Source: CAD feature listing. Evaluate the final solid. Frame: model axes, mm. Face numbers are marked on the shaded views. A direction names the side the tool comes from. Give positions to 0.01 mm unless a question says otherwise; leave off trailing zeros. Write each loop counter-clockwise with the first axis right and the second up, starting at its lowest first coordinate (ties: lowest second). Pieces come first, ordered by that corner, then holes. Notation, with made-up numbers: (86.25, 89) -> (97.25, 89) arc R24 cw to (97.25, 116) -> close; hole circle Ø8 at (72.5, 14.25). An arc over 180 degrees is marked (long way). Answer as a JSON object with one key per item and string values. Group by question number.
Item 1: First-contact query: pin 1 Ø8 at (x, z) = (24.925, -6) entering from -Y; pin 2 Ø2.5 at (y, z) = (-22.225, -93.5) entering from +X; pin 3 Ø1 at (y, z) = (-12.5, -59) entering from +X. Flat tips, straight axial feed; report the tip coordinate or a pass-through.
Item 2: Section query A-A on z = -33.5. Return the cut outline in (x, y) (3 decimals), plus the area to 3 significant figures.
Item 3: Ray query, probe 1 along X at (y, z) = (1.15, -93.5) (3 decimals); probe 2 along Y at (x, z) = (-2.2, -93.5) (3 decimals); probe 3 along X at (y, z) = (-1, -86) (3 decimals). Return the intervals inside material, ascending. Write a range as from..to.
Item 4: Section query D-D on z = -78.5. Return the cut outline in (x, y) (3 decimals).
Item 5: Section query B-B on y = -16.5. Return the cut outline in (x, z) (3 decimals), plus the area to 3 significant figures.
Item 6: Access query for the marked faces 1 and 2. Directions: +Z, -Z, +X, -X, +Y, -Y. A direction counts if a zero-diameter tool reaches every point of the face in a straight line with its end or side. Return the directions, or none.
Item 7: Section query C-C on z = -6. Return the cut outline in (x, y) (3 decimals).
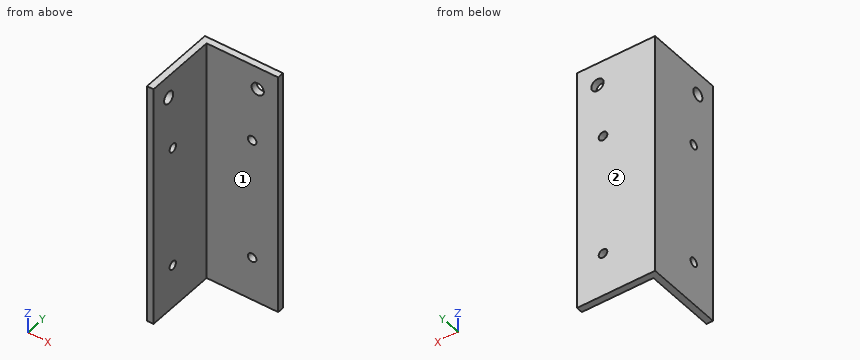
from build123d import *

# Parameters (mm, degrees)
SKETCH1_W                      = 38.1
SKETCH1_H                      = 120
BOSS_EXTRUDE1_DEPTH            = 38.1
SKETCH2_W                      = 34.925
SKETCH2_H                      = 34.925
CUT_EXTRUDE1_DEPTH             = 130.767142413
F_4_2_4_2_DIAMETER_HOLE1_D     = 4.2
F_6_0_6_DIAMETER_HOLE1_D       = 6
F_4_2_4_2_DIAMETER_HOLE2_D     = 4.2
F_4_2_4_2_DIAMETER_HOLE2_DEPTH = 38.1
F_6_0_6_DIAMETER_HOLE2_D       = 6
F_6_0_6_DIAMETER_HOLE2_DEPTH   = 38.1
F_6_0_6_DIAMETER_HOLE3_D       = 6
F_6_0_6_DIAMETER_HOLE3_DEPTH   = 38.1
F_4_2_4_2_DIAMETER_HOLE3_D     = 4.2
SKETCH15_R                     = 2.1
SKETCH15_R_2                   = 3
BOSS_EXTRUDE2_DEPTH            = 3.175
BOSS_EXTRUDE3_START            = -3.175
SKETCH16_R                     = 3
SKETCH16_R_2                   = 2.1
BOSS_EXTRUDE3_DEPTH            = 3.175


with BuildPart() as part:
    # Sketch1 → Boss-Extrude1 (new body)
    with BuildSketch(Plane.XZ.offset(34.925)):
        with Locations((15.875, -55)):
            Rectangle(SKETCH1_W, SKETCH1_H)
    extrude(amount=-BOSS_EXTRUDE1_DEPTH)

    # Sketch2 → Cut-Extrude1 (cut, through all)
    with BuildSketch(Plane(origin=(0, 0, -115), x_dir=(-1, 0, 0), z_dir=(0, 0, -1))):
        with Locations((-17.4625, -17.4625)):
            Rectangle(SKETCH2_W, SKETCH2_H)
    extrude(amount=-CUT_EXTRUDE1_DEPTH, mode=Mode.SUBTRACT)

    # Ø4.2 (4.2) Diameter Hole1 (through all)
    with Locations(Plane(origin=(0, 0, 0), x_dir=(-1, 0, 0), z_dir=(0, -1, 0))):
        with Locations((-5, 35.97), (-5, 91.03)):
            Hole(F_4_2_4_2_DIAMETER_HOLE1_D / 2)

    # Ø6.0 (6) Diameter Hole1 (through all)
    with Locations(Plane(origin=(0, 0, 0), x_dir=(-1, 0, 0), z_dir=(0, -1, 0))):
        with Locations((-22.225, 106.5), (-22.225, 46.5)):
            Hole(F_6_0_6_DIAMETER_HOLE1_D / 2)

    # Ø4.2 (4.2) Diameter Hole2
    with Locations(Plane(origin=(0, 3.175, 0), x_dir=(1, 0, 0), z_dir=(0, 1, 0))):
        with Locations((22.225, 33.5), (22.225, 93.5), (29.296067812, 100.571067812), (29.296067812, 26.428932188)):
            Hole(F_4_2_4_2_DIAMETER_HOLE2_D / 2, depth=F_4_2_4_2_DIAMETER_HOLE2_DEPTH)

    # Ø6.0 (6) Diameter Hole2
    with Locations(Plane(origin=(0, 3.175, 0), x_dir=(1, 0, 0), z_dir=(0, 1, 0))):
        with Locations((24.925, 6)):
            Hole(F_6_0_6_DIAMETER_HOLE2_D / 2, depth=F_6_0_6_DIAMETER_HOLE2_DEPTH)

    # Ø6.0 (6) Diameter Hole3
    with Locations(Plane.ZY.offset(3.175)):
        with Locations((-6, -24.925), (-106.5, -22.225), (-46.5, -22.225)):
            Hole(F_6_0_6_DIAMETER_HOLE3_D / 2, depth=F_6_0_6_DIAMETER_HOLE3_DEPTH)

    # Ø4.2 (4.2) Diameter Hole3 (through all)
    with Locations(Plane.ZY.offset(3.175)):
        with Locations((-93.5, -22.225), (-33.5, -22.225), (-35.97, -5), (-91.03, -5), (-100.571067812, -29.296067812), (-26.428932188, -29.296067812)):
            Hole(F_4_2_4_2_DIAMETER_HOLE3_D / 2)

    # Sketch15 → Boss-Extrude2 (add)
    with BuildSketch(Plane(origin=(0, 3.175, 0), x_dir=(1, 0, 0), z_dir=(0, 1, 0))):
        with Locations((29.296067812, 26.428932188)):
            Circle(SKETCH15_R)
        with Locations((29.296067812, 100.571067812)):
            Circle(SKETCH15_R)
        with Locations((22.225, 106.5)):
            Circle(SKETCH15_R_2)
        with Locations((22.225, 46.5)):
            Circle(SKETCH15_R_2)
        with Locations((5, 35.97)):
            Circle(SKETCH15_R)
        with Locations((5, 91.03)):
            Circle(SKETCH15_R)
    extrude(amount=-BOSS_EXTRUDE2_DEPTH)

    # Sketch16 → Boss-Extrude3 (add)
    with BuildSketch(Plane.ZY.offset(3.175).offset(BOSS_EXTRUDE3_START)):
        with Locations((-106.5, -22.225)):
            Circle(SKETCH16_R)
        with Locations((-100.571067812, -29.296067812)):
            Circle(SKETCH16_R_2)
        with Locations((-46.5, -22.225)):
            Circle(SKETCH16_R)
        with Locations((-26.428932188, -29.296067812)):
            Circle(SKETCH16_R_2)
        with Locations((-35.97, -5)):
            Circle(SKETCH16_R_2)
        with Locations((-91.03, -5)):
            Circle(SKETCH16_R_2)
    extrude(amount=BOSS_EXTRUDE3_DEPTH)


solid = part.part
Worked answers:
{
 "1": {"pin 1": "y = 0", "pin 2": "through", "pin 3": "x = 0"},
 "2": {"outline": "(-3.175, -34.925) -> (0, -34.925) -> (0, -24.325) -> (-3.175, -24.325) -> close; (-3.175, -20.125) -> (0, -20.125) -> (0, 0) -> (20.125, 0) -> (20.125, 3.175) -> (-3.175, 3.175) -> close; (24.325, 0) -> (34.925, 0) -> (34.925, 3.175) -> (24.325, 3.175) -> close", "area": "205 mm^2"},
 "3": {"probe 1": "-3.175..20.125, 24.325..34.925", "probe 2": "-34.925..-24.325, -20.125..3.175", "probe 3": "-3.175..0"},
 "4": {"outline": "(-3.175, -34.925) -> (0, -34.925) -> (0, 0) -> (34.925, 0) -> (34.925, 3.175) -> (-3.175, 3.175) -> close"},
 "5": {"outline": "(-3.175, -115) -> (0, -115) -> (0, 5) -> (-3.175, 5) -> close", "area": "381 mm^2"},
 "6": {"face 1": "+Z, -Z, +X, -Y", "face 2": "+Z, -Z, +X, -X, +Y"},
 "7": {"outline": "(-3.175, -34.925) -> (0, -34.925) -> (0, -27.925) -> (-3.175, -27.925) -> close; (-3.175, -21.925) -> (0, -21.925) -> (0, 0) -> (21.925, 0) -> (21.925, 3.175) -> (-3.175, 3.175) -> close; (27.925, 0) -> (34.925, 0) -> (34.925, 3.175) -> (27.925, 3.175) -> close"}
}
